Geometry check sheet. Reference: the model listing, model coordinates, mm. A direction names the side the tool comes from. Coordinates: 2 decimals unless noted, no trailing zeros. Loops run counter-clockwise (first coordinate to the right, second up) from the corner with the lowest first, then second, coordinate; pieces in that order, holes last. Notation, with made-up numbers: M 10,61.25 L 41,61.25 A26 cw 41,87.25 Z; hole C -20,-22 d4. An arc over 180 degrees is marked long. Use CSV: the item, a comma, the result in double quotes.
Autodesk Inventor part; units mm, degrees
ref_plane "Work Plane1" through (0, 0, 6) normal (0, 0, 1) x (1, 0, 0)
ref_plane "YZ Plane" through (0, 0, 0) normal (1, 0, 0) x (0, 1, 0)
ref_plane "XZ Plane" through (0, 0, 0) normal (0, 1, 0) x (-1, 0, 0)
sketch "Sketch1" plane through (0, 0, 0) normal (0, 0, 1) x (1, 0, 0)
  line L0 (0, 0) -> (0, -15) construction
  line L1 (-5, 0) -> (-5, -15)
  line L2 (5, -15) -> (5, 0)
  arc A0 (5, 0) -> (-5, 0) centre (0, 0) ccw
  arc A1 (-5, -15) -> (5, -15) centre (0, -15) ccw
  line L3 (0, 0) -> (0, -15) construction
  line L4 (-10, 0) -> (-10, -15)
  line L5 (10, -15) -> (10, 0)
  arc A2 (10, 0) -> (-10, 0) centre (0, 0) ccw
  line L6 (0, -15) -> (0, -87) construction
  line L7 (5, -23.6603) -> (5, -82)
  line L8 (-5, -23.6603) -> (-5, -82)
  arc A3 (-10, -15) -> (-5, -23.6603) centre (0, -15) ccw
  arc A4 (5, -23.6603) -> (10, -15) centre (0, -15) ccw
  line L9 (-20, -82) -> (60, -82)
  line L10 (60, -82) -> (60, -87)
  line L11 (60, -87) -> (-20, -87)
  line L12 (-20, -87) -> (-20, -82)
  point P0 (0, -7.5)
  point P1 (0, -7.5)
  dimension "d0" = 15
  dimension "d1" = 5
  dimension "d2" = 10
  dimension "d3" = 72
  dimension "d4" = 5
  dimension "d5" = 5
  dimension "d7" = 80
  dimension "d8" = 5
  dimension "d24" = 15
extrude "Extrusion1" add sketch "Sketch1" along normal blind 12
sketch "Sketch2" plane through (0, 0, 0) normal (0, 0, -1) x (-1, 0, 0)
  arc A0 (-5, -15) -> (5, -15) centre (0, -15) ccw
  line L0 (0, 0) -> (0, -15) construction
  line L1 (-10, 0) -> (-10, -15)
  line L2 (10, -15) -> (10, 0)
  arc A1 (10, 0) -> (-10, 0) centre (0, 0) ccw
  arc A2 (-10, -15) -> (10, -15) centre (0, -15) ccw
  line L3 (0, 0) -> (0, -15) construction
  line L4 (-5, 0) -> (-5, -15)
  line L5 (5, -15) -> (5, 0)
  arc A3 (5, 0) -> (-5, 0) centre (0, 0) ccw
  arc A4 (-5, -15) -> (5, -15) centre (0, -15) ccw
  point P0 (0, -7.5)
  point P1 (0, -7.5)
  point P2 (-5, -15)
  point P3 (5, -15)
  dimension "d11" = 10
  dimension "d12" = 5
extrude "Extrusion2" add sketch "Sketch2" along normal blind 8
sketch "Sketch3" plane through (0, 0, 12) normal (0, 0, 1) x (1, 0, 0)
  line L0 (-20, -82) -> (-20, -87)
  line L1 (-20, -87) -> (60, -87)
  line L2 (-20, -82) -> (60, -82)
  line L3 (60, -82) -> (60, -87)
  line L4 (60, -87) -> (-20, -87)
  line L5 (-20, -87) -> (-20, -82)
  point P0 (0, 0)
  dimension "d23" = 80
extrude "Extrusion3" add sketch "Sketch3" along normal blind 3
ref_plane "Work Plane1" through (0, 0, 6) normal (0, 0, 1) x (1, 0, 0)
sketch "Sketch4" plane through (0, 0, 6) normal (0, 0, 1) x (1, 0, 0)
  arc A0 (-20, -82) -> (-5, -67) centre (-20, -67) ccw
  line L0 (-5, -23.6603) -> (-5, -82)
  line L1 (60, -82) -> (-20, -82)
  line L2 (-5, -67) -> (-20, -67) construction
  line L3 (-20, -67) -> (-20, -82) construction
  line L4 (-20, -82) -> (-5, -82)
  line L5 (-5, -82) -> (-5, -67)
  arc A1 (5, -63) -> (16.8392, -77.6632) centre (20, -63) ccw
  line L6 (5, -82) -> (5, -23.6603)
  line L7 (16.8392, -77.6632) -> (36.9579, -82)
  line L8 (5, -82) -> (5, -63)
  point P0 (0, 0)
  point P1 (-20, -82)
  dimension "d17" = 15
  dimension "d18" = 30
  dimension "d20" = 19
extrude "Extrusion4" add sketch "Sketch4" along normal mid plane 4
properties part number "Stand"
1. Release check for a two-part mould opening along X. For faces 5 (the flat face through (60, -84, 7)), 6 (the cylindrical face through (-9.28, -77.49, 5.97)), 7 (the cylindrical face through (0, 5, 2)) record: +X half, -X half, draft (parallel to the pull), parting line (faces both ways), or undercut.
The answers:
face 5,"+X half"
face 6,"-X half"
face 7,"undercut"
2. Gauge pin test, flat ends, axial feed: P1, Ø10, axis at x = -4, y = -40.5, coming from the +Z side; P2, Ø3, axis at x = 20.5, z = 5, coming from the +Y side; P3, Ø10, axis at y = -61, z = -2, coming from the +X side; P4, Ø9.5, axis at x = 19.5, y = -72.5, coming from the +Z side. Record the tip position at first contact, or that the pin passes through.
The answers:
P1,"z = 12"
P2,"y = -78.13"
P3,"x = 5"
P4,"through"
3. Set-up check for faces 1 (the flat face through (-8, -79, 8)), 2 (the flat face through (5, -52, 6)), 3 (the flat face through (-5, -8, 2)), 4 (the cylindrical face through (0, -25, -4)): record each of +Z, -Z, +X, -X, +Y, -Y from which the full face is reachable in a straight line by a thin tool's end or side.
The answers:
face 1,"+Z, -X"
face 2,"+X"
face 3,"+Z, -Z"
face 4,"-Z, -Y"
4. Section check C-C, the plane x = 0. Record the cut outline in (y, z), plus the area to 3 significant figures.
The answers:
outline,"M -87,0 L -25,0 L -25,-8 L -20,-8 L -20,12 L -82,12 L -82,15 L -87,15 Z; M 5,-8 L 10,-8 L 10,12 L 5,12 Z"
area,"959 mm^2"
5. Section check D-D, the plane z = 6.25. Record the cut outline in (x, y).
The answers:
outline,"M -20,-87 L 60,-87 L 60,-82 L 36.96,-82 L 16.84,-77.66 A15 cw 5,-63 L 5,-23.66 A10 ccw 10,-15 L 10,0 A10 ccw -10,0 L -10,-15 A10 ccw -5,-23.66 L -5,-67 A15 cw -20,-82 Z; hole M -5,-15 A5 ccw 5,-15 L 5,0 A5 ccw -5,0 Z"
6. Section check A-A, the plane y = -11.5. Record the cut outline in (x, z), plus the area to 3 significant figures.
The answers:
outline,"M -10,-8 L -5,-8 L -5,12 L -10,12 Z; M 5,-8 L 10,-8 L 10,12 L 5,12 Z"
area,"200 mm^2"
7. Thickness scan on line 1 (X direction, y = -11.5, z = 5); line 2 (Z direction, x = -2, y = -42); line 3 (Y direction, x = 27, z = 3.25). Record the ranges inside material, lowest first. Write a range as [from, to].
The answers:
line 1,"[-10, -5], [5, 10]"
line 2,"[0, 12]"
line 3,"[-87, -82]"
8. Section check B-B, the plane z = -4. Record the cut outline in (x, y).
The answers:
outline,"M -10,-15 A10 ccw 10,-15 L 10,0 A10 ccw -10,0 Z; hole M -5,-15 A5 ccw 5,-15 L 5,0 A5 ccw -5,0 Z"
